from build123d import *

# Parameters (mm, degrees)
BOSS_EXTRUDE1_DEPTH      = 6.4
SKETCH4_R                = 1.175
BOSS_EXTRUDE2_DEPTH      = 0.25
SKETCH5_R                = 1.175
BOSS_EXTRUDE3_DEPTH      = 0.25
SKETCH6_R                = 1.175
CUT_EXTRUDE1_DEPTH       = 7.9
BOSS_EXTRUDE4_DEPTH      = 1.8
BOSS_EXTRUDE4_DEPTH_BACK = 1.8


with BuildPart() as part:
    # Sketch2 → Boss-Extrude1 (new body)
    with BuildSketch(Plane.XY):
        with BuildLine():
            Line((-7.9, 10.282147184), (-1.391176502, 10.282147184))
            Line((-1.391176502, 10.282147184), (-0.691176502, 9.582147184))
            Line((-0.691176502, 9.582147184), (7.9, 9.582147184))
            ThreePointArc((7.9, 9.582147184), (9.314213562, 8.996360746), (9.9, 7.582147184))
            Line((9.9, 7.582147184), (9.9, 0.082147184))
            Line((9.9, 0.082147184), (6.2, 0.082147184))
            Line((6.2, 0.082147184), (5.8, -0.317852816))
            Line((5.8, -0.317852816), (3.6, -0.317852816))
            Line((3.6, -0.317852816), (3.2, 0.082147184))
            Line((3.2, 0.082147184), (-3.3, 0.082147184))
            Line((-3.3, 0.082147184), (-3.7, -0.317852816))
            Line((-3.7, -0.317852816), (-5.9, -0.317852816))
            Line((-5.9, -0.317852816), (-6.3, 0.082147184))
            Line((-6.3, 0.082147184), (-9.9, 0.082147184))
            Line((-9.9, 0.082147184), (-9.9, 8.282147184))
            ThreePointArc((-9.9, 8.282147184), (-9.314213562, 9.696360746), (-7.9, 10.282147184))
        make_face()
    extrude(amount=BOSS_EXTRUDE1_DEPTH)

    # Sketch4 → Boss-Extrude2 (add)
    with BuildSketch(Plane.XY.offset(6.4)):
        with Locations((-1.8, 1.832147184)):
            Circle(SKETCH4_R)
        with BuildLine():
            Line((-6.3, 2.5), (-6.3, 0.082147184))
            Line((-6.3, 0.082147184), (-5.9, -0.317852816))
            Line((-5.9, -0.317852816), (-3.7, -0.317852816))
            Line((-3.7, -0.317852816), (-3.3, 0.082147184))
            Line((-3.3, 0.082147184), (-3.3, 2.5))
            ThreePointArc((-3.3, 2.5), (-4.8, 4), (-6.3, 2.5))
        make_face()
        with BuildLine():
            Line((3.2, 2.5), (3.2, 0.082147184))
            Line((3.2, 0.082147184), (3.6, -0.317852816))
            Line((3.6, -0.317852816), (5.8, -0.317852816))
            Line((5.8, -0.317852816), (6.2, 0.082147184))
            Line((6.2, 0.082147184), (6.2, 2.5))
            ThreePointArc((6.2, 2.5), (4.7, 4), (3.2, 2.5))
        make_face()
    extrude(amount=BOSS_EXTRUDE2_DEPTH)

    # Sketch5 → Boss-Extrude3 (add)
    with BuildSketch(Plane(origin=(0, 0, 0), x_dir=(-1, 0, 0), z_dir=(0, 0, -1))):
        with Locations((1.8, 1.832147184)):
            Circle(SKETCH5_R)
        with BuildLine():
            Line((6.3, 2.5), (6.3, 0.082147184))
            Line((6.3, 0.082147184), (5.9, -0.317852816))
            Line((5.9, -0.317852816), (3.7, -0.317852816))
            Line((3.7, -0.317852816), (3.3, 0.082147184))
            Line((3.3, 0.082147184), (3.3, 2.5))
            ThreePointArc((3.3, 2.5), (4.8, 4), (6.3, 2.5))
        make_face()
        with BuildLine():
            Line((-3.2, 2.5), (-3.2, 0.082147184))
            Line((-3.2, 0.082147184), (-3.6, -0.317852816))
            Line((-3.6, -0.317852816), (-5.8, -0.317852816))
            Line((-5.8, -0.317852816), (-6.2, 0.082147184))
            Line((-6.2, 0.082147184), (-6.2, 2.5))
            ThreePointArc((-6.2, 2.5), (-4.7, 4), (-3.2, 2.5))
        make_face()
    extrude(amount=BOSS_EXTRUDE3_DEPTH)

    # Sketch6 → Cut-Extrude1 (cut, through all)
    with BuildSketch(Plane.XY.offset(6.65)):
        with Locations((-4.8, 2.5)):
            Circle(SKETCH6_R)
        with Locations((4.7, 2.5)):
            Circle(SKETCH6_R)
    extrude(amount=-CUT_EXTRUDE1_DEPTH, mode=Mode.SUBTRACT)

    # Sketch7 → Boss-Extrude4 (add, two sides)
    with BuildSketch(Plane.XY.offset(3.2)) as boss_extrude4_sk:
        with BuildLine():
            Line((-4.158024121, 10.282147184), (-2.158024121, 10.282147184))
            ThreePointArc((-2.158024121, 10.282147184), (-3.158024121, 11.282147184), (-4.158024121, 10.282147184))
        make_face()
    extrude(amount=BOSS_EXTRUDE4_DEPTH)
    extrude(boss_extrude4_sk.sketch, amount=-BOSS_EXTRUDE4_DEPTH_BACK)


solid = part.part
Geometry: final body of the model. Coordinates: model frame, mm. A direction names the side the tool comes from. Give positions to 0.01 mm unless a question says otherwise; leave off trailing zeros. Write each loop counter-clockwise with the first axis right and the second up, starting at its lowest first coordinate (ties: lowest second). Pieces come first, ordered by that corner, then holes.
(1) Ray query, line 1 (Y direction, x = -4.8, z = 4) (3 decimals); line 2 (X direction, y = 3.25, z = 2.25); line 3 (X direction, y = 1.5, z = 3.5). Return the intervals inside material, ascending.
(2) Cut plane A-A, the plane x = 4.7. Return loops of the section in (y, z) (3 decimals).
(3) Access query for faces 1 (the flat face through (4, 9.582, 3)), 2 (the flat face through (8, 0.082, 3)), 3 (the flat face through (-3, 11, 1.4)). Directions: +Z, -Z, +X, -X, +Y, -Y. A direction counts if a zero-diameter tool reaches every point of the face in a straight line with its end or side. Return the directions, or none.
(4) First-contact query: P1, Ø1.1, axis at x = -8, z = 3.5, coming from the -Y side; P2, Ø1.5, axis at x = 0.5, y = 8.5, coming from the +Z side; P3, Ø0.5, axis at x = -2.5, y = 10.5, coming from the -Z side. Flat tips, straight axial feed; report the tip coordinate or a pass-through.
(5) Mould query, pull axis X, two halves, no side actions, for faces 4 (the cylindrical face through (9.3, 9.01, 3.16)), 5 (the cylindrical face through (3.526, 2.552, 3.248)), 6 (the flat face through (-3, 11, 5)). Classes: released by +X, released by -X, zero draft, split by the parting line, or undercut.
(6) Cut plane B-B, the plane z = 3. Return loops of the section in (x, y) (3 decimals).
(7) Cut plane D-D, the plane x = -4.8. Return loops of the section in (y, z) (3 decimals), then the cut area to 3 significant figures.
(8) Cut plane C-C, the plane x = -1.8. Return loops of the section in (y, z).
Values follow:
1. line 1: y = -0.318 to 1.325, 3.675 to 10.282
1. line 2: x = -9.9 to -5.7, -3.9 to 3.8, 5.6 to 9.9
1. line 3: x = -9.9 to -5.42, -4.18 to 4.08, 5.32 to 9.9
2. outline: (-0.318, -0.25) - (1.325, -0.25) - (1.325, 6.65) - (-0.318, 6.65) - close; (3.675, -0.25) - (4, -0.25) - (4, 0) - (9.582, 0) - (9.582, 6.4) - (4, 6.4) - (4, 6.65) - (3.675, 6.65) - close
3. face 1: +Z, -Z, +X, +Y
3. face 2: +Z, -Z, +X, -Y
3. face 3: -Z, +X, -X, +Y
4. P1: stops at y = 0.08
4. P2: stops at z = 6.4
4. P3: stops at z = 0
5. face 4: released by +X
5. face 5: undercut
5. face 6: zero draft
6. outline: (-9.9, 0.082) - (-6.3, 0.082) - (-5.9, -0.318) - (-3.7, -0.318) - (-3.3, 0.082) - (3.2, 0.082) - (3.6, -0.318) - (5.8, -0.318) - (6.2, 0.082) - (9.9, 0.082) - (9.9, 7.582) arc R2 ccw to (7.9, 9.582) - (-0.691, 9.582) - (-1.391, 10.282) - (-2.158, 10.282) arc R1 ccw to (-4.158, 10.282) - (-7.9, 10.282) arc R2 ccw to (-9.9, 8.282) - close; hole circle Ø2.35 at (-4.8, 2.5); hole circle Ø2.35 at (4.7, 2.5)
7. outline: (-0.318, -0.25) - (1.325, -0.25) - (1.325, 6.65) - (-0.318, 6.65) - close; (3.675, -0.25) - (4, -0.25) - (4, 0) - (10.282, 0) - (10.282, 6.4) - (4, 6.4) - (4, 6.65) - (3.675, 6.65) - close
7. area: 53.8 mm2
8. outline: (0.08, 0) - (0.66, 0) - (0.66, -0.25) - (3.01, -0.25) - (3.01, 0) - (10.28, 0) - (10.28, 6.4) - (3.01, 6.4) - (3.01, 6.65) - (0.66, 6.65) - (0.66, 6.4) - (0.08, 6.4) - close
